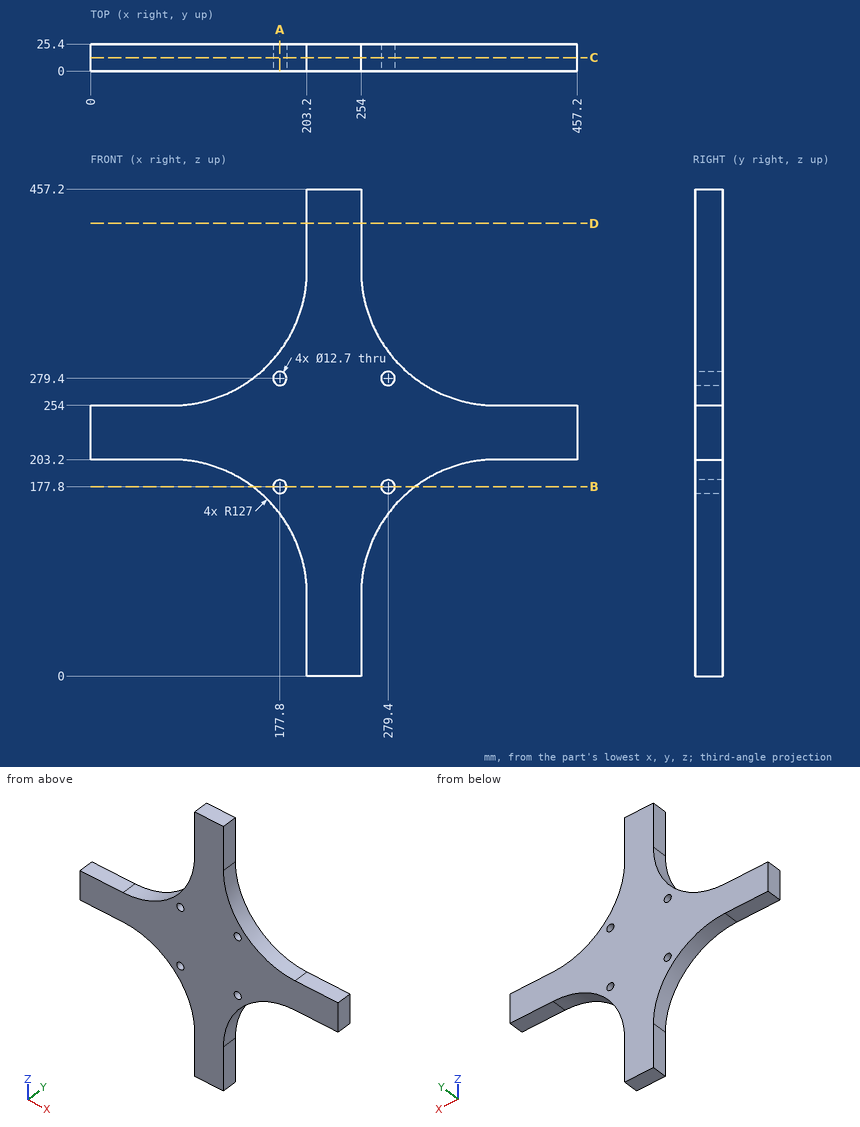
Study the drawing (mm; zero at the part's minimum x, y, z) and answer. Give positions to 0.01 mm unless a question says otherwise; leave off trailing zeros. Write each loop counter-clockwise with the first axis right and the second up, starting at its lowest first coordinate (ties: lowest second). Pieces come first, ordered by that corner, then holes. Notation, with made-up numbers: (42.25, -14) - (69.25, -14) arc R25 cw to (69.25, 0) - close; hole circle Ø7 at (57, -16). An arc over 180 degrees is marked (long way). Write item = value, one per line. Start each with the question number.
Item 1: Each of these flat-tipped pins is pushed along its axis until it touches: P1, Ø2, axis at x = 125, y = 8, coming from the +Z side; P2, Ø12.5, axis at x = 50, y = 16, coming from the +Z side; P3, Ø6, axis at y = 18.5, z = 82, coming from the +X side; P4, Ø7.5, axis at x = 177.8, z = 279.4, coming from the +Y side. Where does it stop, or does it pass through?
Item 2: Find section A-A (x = 177.8). Give the vertices of the cut face in (y, z).
Item 3: Find section B-B (z = 177.8). Give the vertices of the cut face in (x, y).
Item 4: Find the intervals of material crossed by probe 1 along X at (y, z) = (19, 279.4); probe 2 along X at (y, z) = (16, 178), in increasing order. Write a range as [from, to].
Item 5: Find section D-D (z = 425). Give the vertices of the cut face in (x, y), then the cut area to 3 significant figures.
Item 6: Find section C-C (y = 12.5). Give the vertices of the cut face in (x, z), then the cut area to 3 significant figures.
Response:
q1.P1 = 264.17
q1.P2 = 254
q1.P3 = 254.31
q1.P4 = through
q2.outline = (0, 152.4) - (25.4, 152.4) - (25.4, 171.45) - (0, 171.45) - close; (0, 184.15) - (25.4, 184.15) - (25.4, 273.05) - (0, 273.05) - close; (0, 285.75) - (25.4, 285.75) - (25.4, 304.8) - (0, 304.8) - close
q3.outline = (152.4, 0) - (171.45, 0) - (171.45, 25.4) - (152.4, 25.4) - close; (184.15, 0) - (273.05, 0) - (273.05, 25.4) - (184.15, 25.4) - close; (285.75, 0) - (304.8, 0) - (304.8, 25.4) - (285.75, 25.4) - close
q4.probe_1 = [152.4, 171.45], [184.15, 273.05], [285.75, 304.8]
q4.probe_2 = [152.13, 171.45], [184.15, 273.05], [285.75, 305.07]
q5.outline = (203.2, 0) - (254, 0) - (254, 25.4) - (203.2, 25.4) - close
q5.area = 1,290 mm²
q6.outline = (0, 203.2) - (76.2, 203.2) arc R127 cw to (203.2, 76.2) - (203.2, 0) - (254, 0) - (254, 76.2) arc R127 cw to (381, 203.2) - (457.2, 203.2) - (457.2, 254) - (381, 254) arc R127 cw to (254, 381) - (254, 457.2) - (203.2, 457.2) - (203.2, 381) arc R127 cw to (76.2, 254) - (0, 254) - close; hole circle Ø12.7 at (177.8, 177.8); hole circle Ø12.7 at (177.8, 279.4); hole circle Ø12.7 at (279.4, 177.8); hole circle Ø12.7 at (279.4, 279.4)
q6.area = 57,200 mm²
